Read the model definition and answer for the solid it produces. Units are mm, in the model's axes. Give positions to 0.01 mm unless a question says otherwise; leave off trailing zeros. Loops run counter-clockwise (first coordinate to the right, second up) from the corner with the lowest first, then second, coordinate; pieces in that order, holes last. Notation, with made-up numbers: (0, 68.25) -> (58, 68.25) arc R27 ccw to (58, 87.25) -> close; hole circle Ø9 at (11.5, 83.25). An arc over 180 degrees is marked (long way). Write each question's results on one line, items separated by ' | '. Start each with the question number.
Item 1: Section A-A on x = -25 is taken. Write down the section's boundary in (y, z).
Item 2: Section C-C on y = -63 is taken. Write down the section's boundary in (x, z).
Item 3: Find the intervals of material crossed by line 1 (X direction, y = 104.5, z = 1.8); line 2 (Z direction, x = 9.5, y = -7), in increasing order.
Item 4: Section D-D on x = -52 is taken. Write down the section's boundary in (y, z), and give its area (3 significant figures).
Item 5: Section B-B on z = -8.5 is taken. Write down the section's boundary in (x, y), and give its area (3 significant figures).
Item 6: Each of these flat-tipped pins is pushed along its axis until it touches: P1, Ø10, axis at x = -57.5, z = 1, coming from the -Y side; P2, Ø6.5, axis at x = -9.5, z = 4, coming from the -Y side; P3, Ø10, axis at x = 65.5, z = 2, coming from the +Y side. Where does it stop, or does it pass through?
```python
from build123d import *

# Parameters (mm, degrees)
F0_R         = 4
F1_DEPTH     = 6
F3_DEPTH     = 6
F4_R         = 1.5
F5_DEPTH     = 6.001
F6_COUNT     = 4
F8_W         = 85
F8_H         = 12
F9_DEPTH     = 6
F10_R        = 3.55
F10_R_2      = 2.5
F10_W        = 10
F10_H        = 5
F11_DEPTH    = 6.001
F12_C1_SIZE2 = 3
F12_C1_SIZE  = 30
F12_C2_SIZE2 = 30
F12_C2_SIZE  = 3
F12_C3_SIZE2 = 3
F12_C3_SIZE  = 30
F12_C4_SIZE2 = 30
F12_C4_SIZE  = 3
F13_R        = 1
F14_DEPTH    = 20
F15_R        = 3.55
F15_R_2      = 2.5
F16_DEPTH    = 6


# Not quite as in the source:
# - a pattern or mirror of a feature is missing from the dataset's text; its kind, count and spacing are read off the source's solid


with BuildPart() as f1:
    # F0 (on Top) → F1 (new body)
    with BuildSketch(Plane.XY):
        with Locations((-104.5, 104.5)):
            Circle(F0_R)
    extrude(amount=F1_DEPTH)

    # F2 (on Top) → F3 (join, through all)
    with BuildSketch(Plane.XY):
        Polygon((-7.0710678119, 0), (0, 0), (0, 7.0710678119), (-35.3553390593, 42.4264068712), (-100.6362966948, 103.4647238196), (-103.4647238196, 100.6362966948), (-42.4264068712, 35.3553390593), align=None)
    extrude(amount=F3_DEPTH)

    # F4 (on face) → F5 (cut, through all)
    with BuildSketch(Plane.XY.offset(6)):
        with Locations((-104.5, 104.5)):
            Circle(F4_R)
    extrude(amount=-F5_DEPTH, mode=Mode.SUBTRACT)


with BuildPart() as f6_1:
    # F6: instance of F1
    add(f1.part.rotate(Axis((0, 0, 3), (0, 0, -1)), 1 * 360 / F6_COUNT))


with BuildPart() as f6_2:
    # F6: instance of F1
    add(f1.part.rotate(Axis((0, 0, 3), (0, 0, -1)), 2 * 360 / F6_COUNT))


with BuildPart() as f6_3:
    # F6: instance of F1
    add(f1.part.rotate(Axis((0, 0, 3), (0, 0, -1)), 3 * 360 / F6_COUNT))


with BuildPart() as f1_1:
    add(f1.part)

    # F7: union F6_1, F6_2, F6_3
    add(f6_1.part)
    add(f6_2.part)
    add(f6_3.part)

    # F8 (on Top) → F9 (join, through all)
    with BuildSketch(Plane.XY):
        with Locations((0, 42.5)):
            Rectangle(F8_W, F8_H)
    f9 = extrude(amount=F9_DEPTH)

    # F9_copies: F9 across plane
    add(f9.mirror(Plane(origin=(0, 0, 0), x_dir=(0, 0, -1), z_dir=(0, -1, 0))))

    # F10 (on face) → F11 (cut, through all)
    with BuildSketch(Plane.XY.offset(6)):
        with Locations((-21, 42.5)):
            Circle(F10_R)
        with Locations((21, 42.5)):
            Circle(F10_R_2)
        with Locations((0, 43)):
            Rectangle(F10_W, F10_H)
    f11 = extrude(amount=-F11_DEPTH, mode=Mode.SUBTRACT)

    # F11_copies: F11 across plane
    add(f11.mirror(Plane(origin=(0, 0, 0), x_dir=(0, 0, -1), z_dir=(0, -1, 0))), mode=Mode.SUBTRACT)

    # F12: chamfer of 3 x 30 on 4 edges, made by hand

    # F12_c1
    f12_c1_edges = [f1_1.edges().sort_by_distance(p)[0] for p in [
        (-41.8510944399, 48.5, 3),
    ]]
    f12_c1_side = f1_1.faces().sort_by_distance((-41.8949210948, 48.5409783396, 3))[0]
    chamfer(f12_c1_edges, length=F12_C1_SIZE, length2=F12_C1_SIZE2, reference=f12_c1_side)

    # F12_c2
    f12_c2_edges = [f1_1.edges().sort_by_distance(p)[0] for p in [
        (41.8510944399, 48.5, 3),
    ]]
    f12_c2_side = f1_1.faces().sort_by_distance((41.7910944399, 48.5, 3))[0]
    chamfer(f12_c2_edges, length=F12_C2_SIZE, length2=F12_C2_SIZE2, reference=f12_c2_side)

    # F12_c3
    f12_c3_edges = [f1_1.edges().sort_by_distance(p)[0] for p in [
        (41.8510944399, -48.5, 3),
    ]]
    f12_c3_side = f1_1.faces().sort_by_distance((41.8949210948, -48.5409783396, 3))[0]
    chamfer(f12_c3_edges, length=F12_C3_SIZE, length2=F12_C3_SIZE2, reference=f12_c3_side)

    # F12_c4
    f12_c4_edges = [f1_1.edges().sort_by_distance(p)[0] for p in [
        (-41.8510944399, -48.5, 3),
    ]]
    f12_c4_side = f1_1.faces().sort_by_distance((-41.7910944399, -48.5, 3))[0]
    chamfer(f12_c4_edges, length=F12_C4_SIZE, length2=F12_C4_SIZE2, reference=f12_c4_side)



with BuildPart() as f14:
    # F13 (on Top) → F14 (new body)
    with BuildSketch(Plane.XY):
        with Locations((-21, 42.5)):
            Circle(F13_R)
    extrude(amount=-F14_DEPTH)


with BuildPart() as f14b:
    # F13 (on Top) → F14, piece 2 (new body)
    with BuildSketch(Plane.XY):
        with Locations((21, 42.5)):
            Circle(F13_R)
    extrude(amount=-F14_DEPTH)


with BuildPart() as f14c:
    # F13 (on Top) → F14, piece 3 (new body)
    with BuildSketch(Plane.XY):
        with Locations((-21, -42.5)):
            Circle(F13_R)
    extrude(amount=-F14_DEPTH)


with BuildPart() as f14d:
    # F13 (on Top) → F14, piece 4 (new body)
    with BuildSketch(Plane.XY):
        with Locations((21, -42.5)):
            Circle(F13_R)
    extrude(amount=-F14_DEPTH)


with BuildPart() as f1_2:
    add(f1_1.part)

    add(f14.part)  # F16 merges F14

    add(f14b.part)  # F16 merges F14b

    add(f14c.part)  # F16 merges F14c

    add(f14d.part)  # F16 merges F14d
    # F15 (on face) → F16 (join)
    with BuildSketch(Plane.XY.offset(6)):
        with Locations((-21, -42.5)):
            Circle(F15_R)
        with Locations((21, -42.5)):
            Circle(F15_R_2)
        with Locations((21, 42.5)):
            Circle(F15_R_2)
        with Locations((-21, 42.5)):
            Circle(F15_R)
    extrude(amount=-F16_DEPTH)


solid = f1_2.part
```
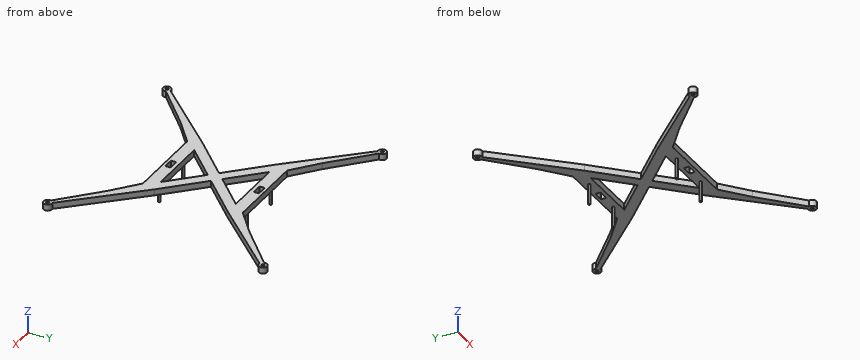
Findings:
1) outline: (-48.5, 0) -> (-36.5, 0) -> (-36.5, 6) -> (-48.5, 6) -> close; (-32.07, 0) -> (-17.93, 0) -> (-17.93, 6) -> (-32.07, 6) -> close; (17.93, 0) -> (32.07, 0) -> (32.07, 6) -> (17.93, 6) -> close; (36.5, 0) -> (48.5, 0) -> (48.5, 6) -> (36.5, 6) -> close
2) outline: (-68.27, 0) -> (-56.48, 0) -> (-56.48, 6) -> (-68.27, 6) -> close; (56.48, 0) -> (68.27, 0) -> (68.27, 6) -> (56.48, 6) -> close
3) line 1: -108.5 to -106, -103 to -100.5, 100.5 to 103, 106 to 108.5 | line 2: 0 to 6
4) outline: (-59.31, 0) -> (-45.59, 0) -> (-45.59, 6) -> (-59.31, 6) -> close; (45.59, 0) -> (59.31, 0) -> (59.31, 6) -> (45.59, 6) -> close | area: 165 mm2
5) outline: circle Ø2 at (-21, -42.5); circle Ø2 at (-21, 42.5); circle Ø2 at (21, -42.5); circle Ø2 at (21, 42.5) | area: 12.6 mm2
6) P1: y = -67.95 | P2: y = -48.5 | P3: y = 75.29
